```python
from build123d import *

# Parameters (mm, degrees)
SKETCH_1_R         = 1.65
SKETCH_1_R_2       = 5.5
EXTRUDE_2450_DEPTH = 2
FILLET_1_R         = 2


with BuildPart() as part:
    # Эскиз1 → Extrude 2450 (new body)
    with BuildSketch(Plane(origin=(0, 0, 0), x_dir=(1, 0, 0), z_dir=(0, 1, 0))):
        with BuildLine():
            Line((-11.508257905, 3.4), (-25.414069539, 7.508333333))
            ThreePointArc((-25.414069539, 7.508333333), (-18.086736192, 19.368014197), (-5.754049101, 25.86775829))
            ThreePointArc((-5.754049101, 25.86775829), (8.055154344, 25.246078676), (19.6725691, 17.755))
            Line((19.6725691, 17.755), (44.541665887, -9.8))
            ThreePointArc((44.541665887, -9.8), (53.912240119, -23.666174502), (59.088465181, -39.58110934))
            ThreePointArc((59.088465181, -39.58110934), (54.221507729, -46.531844924), (47.270772145, -41.664887472))
            ThreePointArc((47.270772145, -41.664887472), (35.068418794, -17.224917951), (11.508257905, -3.4))
            ThreePointArc((11.508257905, -3.4), (-3.4, -11.508257905), (-11.508257905, 3.4))
        make_face()
        with Locations(Location((-5.785088487, 6.894399988, 0), (0, 0, 270))):
            Circle(SKETCH_1_R, mode=Mode.SUBTRACT)
        with Locations(Location((8.863269777, 1.562833599, 0), (0, 0, 270))):
            Circle(SKETCH_1_R, mode=Mode.SUBTRACT)
        with Locations(Location((0, 0, 0), (0, 0, 270))):
            Circle(SKETCH_1_R_2, mode=Mode.SUBTRACT)
        with Locations(Location((-3.07818129, -8.457233587, 0), (0, 0, 270))):
            Circle(SKETCH_1_R, mode=Mode.SUBTRACT)
        with Locations(Location((-19.513769828, 12.174267415, 0), (0, 0, 270))):
            Circle(SKETCH_1_R, mode=Mode.SUBTRACT)
        with Locations(Location((-10.812286687, 20.300109768, 0), (0, 0, 90))):
            Circle(SKETCH_1_R, mode=Mode.SUBTRACT)
        with Locations(Location((53.179618663, -40.622998406, 0), (0, 0, 270))):
            Circle(SKETCH_1_R, mode=Mode.SUBTRACT)
        with Locations(Location((46.765371804, -23, 0), (0, 0, 270))):
            Circle(SKETCH_1_R, mode=Mode.SUBTRACT)
        with Locations(Location((34.710530923, -8.633600072, 0), (0, 0, 270))):
            Circle(SKETCH_1_R, mode=Mode.SUBTRACT)
    extrude(amount=EXTRUDE_2450_DEPTH)

    # Скругление1
    fillet_1_edges = [part.edges().sort_by_distance(p)[0] for p in [
        (11.508257905, 1, 3.4),
    ]]
    fillet(fillet_1_edges, radius=FILLET_1_R)


solid = part.part
```
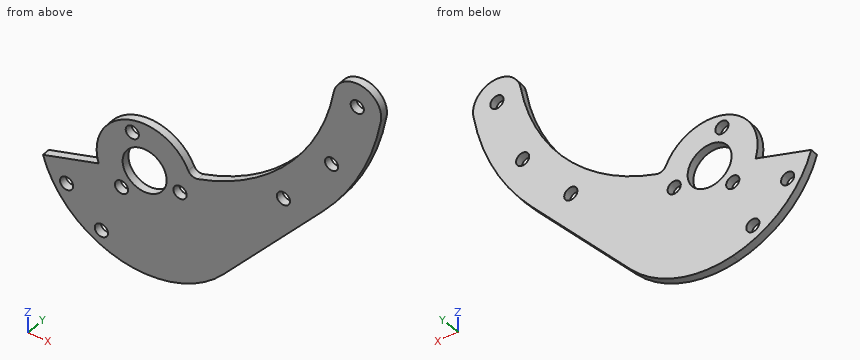
The model under review builds one solid part; all positions refer to its coordinate system, in mm. Coordinates: 2 decimals unless noted, no trailing zeros. Write each loop counter-clockwise with the first axis right and the second up, starting at its lowest first coordinate (ties: lowest second). Pieces come first, ordered by that corner, then holes. Notation, with made-up numbers: (-3, -37) - (45, -37) arc R34 ccw to (45, 0) - close; hole circle Ø2 at (-8.75, 12.5). An arc over 180 degrees is marked (long way). Answer in a Markdown table with one row per item. Add a question column.
Q1. Consider section B-B on z = 23. Give the boundary of the cut face in (x, y), then the cut area to 3 significant figures.
Q2. Clearance check with flat-ended pins moving along their axes: pin 1 (4.5 mm diameter, centred on x = 8.86, z = -1.56, fed in from +Y); pin 2 (2 mm diameter, centred on x = 46.77, z = 23, fed in from -Y); pin 3 (1 mm diameter, centred on x = 33, y = 0.5, fed in from +Z). State where each tip first meets the part, or that it passes through.
Q3. Consider section D-D on y = 0.7. Give the number of separate pieces and of enclosed holes in the cut face, then the cut area to 3 significant figures.
Q4. Consider section A-A on x = 0. Give the boundary of the cut face in (y, z), then the cut area to 3 significant figures.
Q5. To check wall thickness, follow line 1 along Z through (x, y) = (-5, 1.95); line 2 along X through (y, z) = (0.75, -1.5); line 3 along Z through (x, y) = (-10.5, 0.8). State the ranges of each line that lie inside material, in increasing order. Write a range as from..to.
Q6. Consider section C-C on z = -15. Give the boundary of the cut face in (x, y).
Answers below:
| question | item | result |
|---|---|---|
| 1 | outline | (39.69, 0) - (45.12, 0) - (45.12, 2) - (39.69, 2) - close; (48.42, 0) - (53.58, 0) - (53.58, 2) - (48.42, 2) - close |
| 1 | area | 21.2 mm² |
| 2 | pin 1 | y = 2 |
| 2 | pin 2 | through |
| 2 | pin 3 | z = 15.62 |
| 3 | separate pieces | 1 |
| 3 | enclosed holes | 9 |
| 3 | area | 1,860 mm² |
| 4 | outline | (0, -26.5) - (2, -26.5) - (2, -5.5) - (0, -5.5) - close; (0, 5.5) - (2, 5.5) - (2, 12) - (0, 12) - close |
| 4 | area | 55.0 mm² |
| 5 | line 1 | -26.02..-8.35, -5.44..-2.29, 2.29..10.91 |
| 5 | line 2 | -11.91..-5.29, 5.29..7.21, 10.51..34.34 |
| 5 | line 3 | -24.33..-21.92, -18.68..5.81 |
| 6 | outline | (-21.85, 0) - (22.16, 0) - (22.16, 2) - (-21.85, 2) - close |
